Autodesk Inventor part; units mm, degrees
ref_plane "YZ Plane" through (0, 0, 0) normal (1, 0, 0) x (0, 1, 0)
ref_plane "XZ Plane" through (0, 0, 0) normal (0, 1, 0) x (-1, 0, 0)
ref_plane "XY Plane" through (0, 0, 0) normal (0, 0, 1) x (1, 0, 0)
sketch "Sketch1" plane through (0, 0, 0) normal (1, 0, 0) x (0, 1, 0)
  line L0 (0, 0) -> (0, -0.75) construction
  line L1 (0, 0) -> (0, 0.75) construction
  line L2 (0, 0.75) -> (11, 0.75)
  line L3 (11, 0.75) -> (11, 2.45)
  line L4 (0, -0.75) -> (11, -0.75)
  line L5 (11, -0.75) -> (11, -2.45)
  line L6 (0, 0.75) -> (0, 2.75)
  line L7 (0, 2.75) -> (11, 2.45)
  line L8 (0, -0.75) -> (0, -2.75)
  line L9 (0, -2.75) -> (11, -2.45)
  line L10 (0, -0.75) -> (0, 0.75)
  line L11 (0, 2.75) -> (0, 10.75)
  line L12 (0, -2.75) -> (0, -10.75)
  line L13 (0, -2.75) -> (8, -2.75) construction
  line L14 (0, -10.75) -> (-1.2, -10.75)
  line L15 (-1.2, -10.75) -> (-1.2, 10.75)
  line L16 (-1.2, 10.75) -> (0, 10.75)
  dimension "d0" = 0.75
  dimension "d1" = 0.75
  dimension "d2" = 11
  dimension "d3" = 1.7
  dimension "d4" = 11
  dimension "d5" = 1.7
  dimension "d6" = 2
  dimension "d7" = 2
  dimension "d8" = 8
  dimension "d9" = 8
  dimension "d10" = 90
  dimension "d11" = 1.2
extrude "Extrusion1" add sketch "Sketch1" along normal blind 35
fillet "Fillet1" radius 3.5875 2 edges at (17.5, 0, 2.75) (17.5, 0, -2.75)
fillet "Fillet2" radius 2 2 edges at (17.5, 0, 10.75) (17.5, 0, -10.75)
properties part number "cleat bracket v1"
Input: part model. Units: mm. Frame: model coordinates. A direction names the side the tool comes from. Give positions to 0.01 mm unless a question says otherwise; leave off trailing zeros. Order: outer loops, then holes, each group sorted by start corner. A loop starts at its lowest first (then second) coordinate and runs counter-clockwise, first axis right, second up. Notation, with made-up numbers: M 30.25,24 L 72.25,24 A24 cw 72.25,40 Z; hole C 64.5,71 d2. An arc over 180 degrees is marked long. Return JSON: item names as keys, results as strings.
1) Contact query for flat-ended pins moving along their axis: pin 1 (1.5 mm diameter, centred on x = 8.5, y = 0.5, fed in from -Z); pin 2 (5 mm diameter, centred on x = 24, z = -6.5, fed in from +Y); pin 3 (6 mm diameter, centred on x = 4.5, y = 7, fed in from -Z). Output: stop coordinate, or through.
Taken from the geometry:
{"pin 1": "stops at z = -9.89", "pin 2": "stops at y = 0.79", "pin 3": "stops at z = -2.64"}
2) Access query for faces 4 (the face through (35, 2, 1)), 5 (the face through (17, 0, -8)), 6 (the face through (17, 5, -0.75)), 7 (the face through (17, -1.2, 0)), 8 (the face through (17, 0, 8)). Directions: +Z, -Z, +X, -X, +Y, -Y. A direction counts if a zero-diameter tool reaches every point of the face in a straight line with its end or side. Return the directions, or none.
Taken from the geometry:
{"face 4": "+Z, -Z, +X, +Y, -Y", "face 5": "-Z, +X, -X, +Y", "face 6": "+X, -X, +Y", "face 7": "+Z, -Z, +X, -X, -Y", "face 8": "+Z, +X, -X, +Y"}
3) Section query C-C on y = 10.5. Output: boundary loops of the cut face in (x, z), and give its area (3 significant figures).
Taken from the geometry:
{"outline": "M 0,-2.46 L 35,-2.46 L 35,-0.75 L 0,-0.75 Z; M 0,0.75 L 35,0.75 L 35,2.46 L 0,2.46 Z", "area": "120 mm2"}
4) Section query A-A on y = 2. Output: boundary loops of the cut face in (x, z), and give its area (3 significant figures).
Taken from the geometry:
{"outline": "M 0,-3.02 L 35,-3.02 L 35,-0.75 L 0,-0.75 Z; M 0,0.75 L 35,0.75 L 35,3.02 L 0,3.02 Z", "area": "159 mm2"}
5) Line query: L1, parallel to Z at x = 14.5, y = 3.75; L2, parallel to Y at x = 25, z = -8; L3, parallel to Z at x = 13, y = 8.75. Output: solid intervals per line, ascending. Write a range as [from, to].
Taken from the geometry:
{"L1": "z = [-2.65, -0.75], [0.75, 2.65]", "L2": "y = [-1.2, 0]", "L3": "z = [-2.51, -0.75], [0.75, 2.51]"}
6) Section query D-D on z = -0.25. Output: boundary loops of the cut face in (x, y), and give its area (3 significant figures).
Taken from the geometry:
{"outline": "M 0,-1.2 L 35,-1.2 L 35,0 L 0,0 Z", "area": "42.0 mm2"}
7) Mould query, pull axis Z, two halves, no side actions, for faces 1 (the face through (17.26, -0.34, 10.03)), 2 (the face through (17, 5, 0.75)), 3 (the face through (0, 2, 1)). Classes: released by +Z, released by -Z, zero draft, split by the parting line, or undercut.
Taken from the geometry:
{"face 1": "released by +Z", "face 2": "undercut", "face 3": "zero draft"}
